Design review of the part built by this model. Coordinates are the model's own, in mm. Coordinates: 2 decimals unless noted, no trailing zeros. Write each loop counter-clockwise with the first axis right and the second up, starting at its lowest first coordinate (ties: lowest second). Pieces come first, ordered by that corner, then holes. Notation, with made-up numbers: (72, 22.5) - (78, 22.5) arc R30 ccw to (78, 51.5) - close; hole circle Ø1 at (-5.5, -13.5). An arc over 180 degrees is marked (long way). Use a Markdown table: item, result.
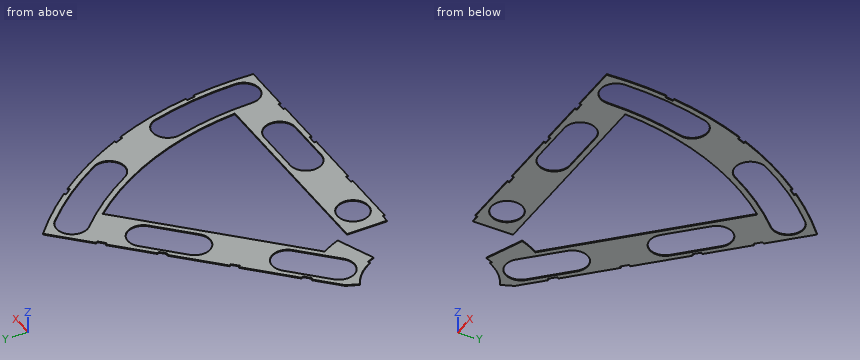
from build123d import *

# Parameters (mm, degrees)
BOSS_EXTRUDE1_DEPTH = 0.254
SKETCH2_R           = 4.699
CUT_EXTRUDE1_DEPTH  = 1.254
SKETCH3_W           = 2.54
SKETCH3_H           = 0.635
CUT_EXTRUDE2_DEPTH  = 1.254
CUT_EXTRUDE4_DEPTH  = 1.254
CUT_EXTRUDE5_DEPTH  = 1.254


with BuildPart() as part:
    # Sketch1 → Boss-Extrude1 (new body)
    with BuildSketch(Plane.XY):
        with BuildLine():
            Line((67.21146711, 76.191723231), (8.696654013, 17.676910134))
            Line((8.696654013, 17.676910134), (7.228954972, 14.133571205))
            ThreePointArc((7.228954972, 14.133571205), (14.666587579, 6.075099489), (15.105587123, -4.88230096))
            Line((15.105587123, -4.88230096), (18.648926052, -6.35))
            Line((18.648926052, -6.35), (101.401368334, -6.35))
            ThreePointArc((101.401368334, -6.35), (93.866160503, 38.880636728), (67.21146711, 76.191723231))
        make_face()
        with BuildLine():
            Line((88.672924278, 6.35), (27.86051193, 6.35))
            ThreePointArc((27.86051193, 6.35), (26.399857642, 10.93517908), (24.190484974, 15.210228852))
            Line((24.190484974, 15.210228852), (67.191354125, 58.211098004))
            ThreePointArc((67.191354125, 58.211098004), (82.13289044, 34.020557137), (88.672924278, 6.35))
        make_face(mode=Mode.SUBTRACT)
    extrude(amount=BOSS_EXTRUDE1_DEPTH)

    # Sketch2 → Cut-Extrude1 (cut, through all)
    with BuildSketch(Plane.XY.offset(0.254)):
        with Locations((22.225, 0)):
            Circle(SKETCH2_R)
        with Locations((36.195, 0)):
            Circle(SKETCH2_R)
        with Locations((61.722, 0)):
            Circle(SKETCH2_R)
        with Locations((75.692, 0)):
            Circle(SKETCH2_R)
        with Locations((95.25, 0)):
            Circle(SKETCH2_R)
        with Locations((15.715448212, 15.715448212)):
            Circle(SKETCH2_R)
        with Locations((25.593729945, 25.593729945)):
            Circle(SKETCH2_R)
        with Locations((43.644044748, 43.644044748)):
            Circle(SKETCH2_R)
        with Locations((53.522326482, 53.522326482)):
            Circle(SKETCH2_R)
        with Locations((92.004434954, 24.652514046)):
            Circle(SKETCH2_R)
        with Locations((82.48891971, 47.625)):
            Circle(SKETCH2_R)
        with Locations((67.351920908, 67.351920908)):
            Circle(SKETCH2_R)
    extrude(amount=-CUT_EXTRUDE1_DEPTH, mode=Mode.SUBTRACT)

    # Sketch3 → Cut-Extrude2 (cut, through all)
    with BuildSketch(Plane.XY.offset(0.254)):
        Polygon((15.266435406, 24.246691527), (17.06248663, 26.042742751), (17.511499436, 25.593729945), (15.715448212, 23.797678721), align=None)
        Polygon((44.991083167, 53.971339288), (43.195031942, 52.175288063), (43.644044748, 51.726275257), (45.440095973, 53.522326482), align=None)
        with Locations((29.21, -6.0325)):
            Rectangle(SKETCH3_W, SKETCH3_H)
        with Locations((68.707, -6.0325)):
            Rectangle(SKETCH3_W, SKETCH3_H)
        Polygon((29.230733674, 38.210989795), (31.026784898, 40.007041019), (31.475797704, 39.558028213), (29.67974648, 37.761976989), align=None)
        Polygon((56.845021246, 65.825277367), (55.048970022, 64.029226143), (55.497982828, 63.580213337), (57.294034052, 65.376264561), align=None)
        with Locations((48.9585, -6.0325)):
            Rectangle(SKETCH3_W, SKETCH3_H)
        with Locations((85.471, -6.0325)):
            Rectangle(SKETCH3_W, SKETCH3_H)
        Polygon((99.935462164, 14.437711971), (100.266998693, 11.919442024), (101.526133667, 12.085210288), (101.194597138, 14.603480236), align=None)
        Polygon((93.765504959, 37.464305742), (94.938831965, 37.950313702), (93.966816047, 40.296967714), (92.793489041, 39.810959755), align=None)
        Polygon((79.327792988, 62.471156422), (80.874047017, 60.456038938), (81.88160576, 61.229165953), (80.33535173, 63.244283437), align=None)
        Polygon((13.593916116, 7.005422516), (14.565932035, 4.658768503), (15.739259041, 5.144776462), (14.767243123, 7.491430475), align=None)
    extrude(amount=-CUT_EXTRUDE2_DEPTH, mode=Mode.SUBTRACT)

    # Sketch6 → Cut-Extrude4 (cut, through all)
    with BuildSketch(Plane.XY.offset(0.254)):
        with BuildLine():
            Line((12.392753447, 19.038142977), (22.27103518, 28.91642471))
            ThreePointArc((22.27103518, 28.91642471), (28.91642471, 28.91642471), (28.91642471, 22.27103518))
            Line((28.91642471, 22.27103518), (19.038142977, 12.392753447))
            ThreePointArc((19.038142977, 12.392753447), (12.392753447, 12.392753447), (12.392753447, 19.038142977))
        make_face()
        with BuildLine():
            Line((40.321349984, 46.966739513), (50.199631717, 56.845021246))
            ThreePointArc((50.199631717, 56.845021246), (56.845021246, 56.845021246), (56.845021246, 50.199631717))
            Line((56.845021246, 50.199631717), (46.966739513, 40.321349984))
            ThreePointArc((46.966739513, 40.321349984), (40.321349984, 40.321349984), (40.321349984, 46.966739513))
        make_face()
        with BuildLine():
            Line((61.722, 4.699), (75.692, 4.699))
            ThreePointArc((75.692, 4.699), (80.391, 0), (75.692, -4.699))
            Line((75.692, -4.699), (61.722, -4.699))
            ThreePointArc((61.722, -4.699), (57.023, 0), (61.722, 4.699))
        make_face()
        with BuildLine():
            ThreePointArc((99.949, 0), (99.093922449, 13.045962386), (96.543320412, 25.868704739))
            ThreePointArc((96.543320412, 25.868704739), (90.788244261, 29.191399504), (87.465549496, 23.436323353))
            ThreePointArc((87.465549496, 23.436323353), (89.776323642, 11.819277232), (90.551, 0))
            ThreePointArc((90.551, 0), (95.25, -4.699), (99.949, 0))
        make_face()
        with BuildLine():
            ThreePointArc((86.558373083, 49.9745), (79.294873009, 60.845096068), (70.674615673, 70.674615673))
            ThreePointArc((70.674615673, 70.674615673), (64.029226143, 70.674615673), (64.029226143, 64.029226143))
            ThreePointArc((64.029226143, 64.029226143), (71.838938317, 55.123956158), (78.419466338, 45.2755))
            ThreePointArc((78.419466338, 45.2755), (84.83841971, 43.555546628), (86.558373083, 49.9745))
        make_face()
    extrude(amount=-CUT_EXTRUDE4_DEPTH, mode=Mode.SUBTRACT)

    # Sketch5 → Cut-Extrude5 (cut, through all)
    with BuildSketch(Plane.XY.offset(0.254)):
        Polygon((11.640421912, 3.584446343), (28.067, 10.38855777), (28.067, -7.62), (11.640421912, -7.62), align=None)
    extrude(amount=-CUT_EXTRUDE5_DEPTH, mode=Mode.SUBTRACT)


solid = part.part
(1) For L1, parallel to Y at x = 74.5, z = 0.15; L2, parallel to X at y = 49, z = 0.2; L3, parallel to X at y = 8, z = 0.15, list the stretches that pass through material, from the lowest coordinate up. Write a range as from..to.
Determined:
| item | result |
|---|---|
| L1 | -6.35..-4.7, 4.7..6.35, 48.51..51.47, 66.63..69.08 |
| L2 | 40.02..42.35, 55.65..57.98, 74.18..76.15, 86.98..89 |
| L3 | 13.71..22.3, 88.54..90.2, 99.63..101.28 |
(2) Take a section at A-A on y = 41.5. Write out the cut boundary in (x, z).
Determined:
| item | result |
|---|---|
| outline | (32.52, 0) - (39.46, 0) - (39.46, 0.25) - (32.52, 0.25) - close; (48.15, 0) - (50.48, 0) - (50.48, 0.25) - (48.15, 0.25) - close; (78.62, 0) - (92.74, 0) - (92.74, 0.25) - (78.62, 0.25) - close |
(3) Take a section at B-B on x = 32.5. Write out the cut boundary in (y, z).
Determined:
| item | result |
|---|---|
| outline | (-6.35, 0) - (-2.9, 0) - (-2.9, 0.25) - (-6.35, 0.25) - close; (2.9, 0) - (6.35, 0) - (6.35, 0.25) - (2.9, 0.25) - close; (23.52, 0) - (41.48, 0) - (41.48, 0.25) - (23.52, 0.25) - close |
(4) Take a section at C-C on z = 0.15. State how many separate pieces and enclosed holes the cut face has, and give its area (3 significant figures).
Determined:
| item | result |
|---|---|
| separate pieces | 1 |
| enclosed holes | 6 |
| area | 1,560 mm2 |
